```python
from build123d import *

# Parameters (mm, degrees)
F0_R     = 2.5
F1_DEPTH = 5
F2_SIZE  = 4.99999


# Not quite as in the source:
# - a fillet or chamfer is up to 0.001 mm smaller than in the source, because OpenCascade refuses the exact size


with BuildPart() as f1:
    # F0 (on Top) → F1 (new body)
    with BuildSketch(Plane.XY):
        with BuildLine():
            ThreePointArc((100, 15), (97.0710678119, 22.0710678119), (90, 25))
            Line((90, 25), (-90, 25))
            ThreePointArc((-90, 25), (-97.0710678119, 22.0710678119), (-100, 15))
            Line((-100, 15), (-100, -15))
            ThreePointArc((-100, -15), (-97.0710678119, -22.0710678119), (-90, -25))
            Line((-90, -25), (90, -25))
            ThreePointArc((90, -25), (97.0710678119, -22.0710678119), (100, -15))
            Line((100, -15), (100, 15))
        make_face()
        with Locations((-50, 0)):
            Circle(F0_R, mode=Mode.SUBTRACT)
        with Locations((50, 0)):
            Circle(F0_R, mode=Mode.SUBTRACT)
    extrude(amount=F1_DEPTH)

    # F2 (size 5 in the source; OpenCascade refuses exactly that, so slightly less here)
    f2_edges = [f1.edges().sort_by_distance(p)[0] for p in [
        (-52.5, 0, 0),
        (47.5, 0, 0),
    ]]
    chamfer(f2_edges, length=F2_SIZE)


solid = f1.part
```
Source: CAD feature listing. Evaluate the final solid. Frame: model axes, mm. Round coordinates to 2 decimals unless told otherwise and drop trailing zeros. Loops run counter-clockwise (first coordinate to the right, second up) from the corner with the lowest first, then second, coordinate; pieces in that order, holes last. Notation, with made-up numbers: M -36,-11 L 6,-11 A29 cw 6,10 Z; hole C -31.75,-2 d2. An arc over 180 degrees is marked long. Use a Markdown table: item, result. Add a question column.
1. Ray query, line 1 along X through (y, z) = (3, 3.1); line 2 along X through (y, z) = (-4.5, 1.75); line 3 along X through (y, z) = (21.5, 4.8). Return the intervals inside material, ascending. Write a range as [from, to].
2. Cut plane D-D, the plane y = 21. Output: boundary loops of the cut face in (x, z), and give its area (3 significant figures).
3. Pull-direction query (X, two-part tool) for faces 1 (the conical face through (52.68, 0.84, 4.69)), 2 (the flat face through (100, 0, 2)), 3 (the flat face through (-1, 0, 5)); classes: +X half, -X half, draft (parallel to the pull), parting line (faces both ways), or undercut.
4. Cut plane C-C, the plane y = 0. State how many separate pieces and enclosed holes the cut face has, and give its area (3 significant figures).
5. Cut plane B-B, the plane z = 3.45. Output: boundary loops of the cut face in (x, y), and give its area (3 significant figures).
Solution:
| question | item | result |
|---|---|---|
| 1 | line 1 | x = [-100, -53.22], [-46.78, 46.78], [53.22, 100] |
| 1 | line 2 | x = [-100, -53.58], [-46.42, 46.42], [53.58, 100] |
| 1 | line 3 | x = [-97.6, 97.6] |
| 2 | outline | M -98,0 L 98,0 L 98,5 L -98,5 Z |
| 2 | area | 980 mm2 |
| 3 | face 1 | undercut |
| 3 | face 2 | +X half |
| 3 | face 3 | draft |
| 4 | separate pieces | 3 |
| 4 | enclosed holes | 0 |
| 4 | area | 900 mm2 |
| 5 | outline | M -100,-15 A10 ccw -90,-25 L 90,-25 A10 ccw 100,-15 L 100,15 A10 ccw 90,25 L -90,25 A10 ccw -100,15 Z; hole C -50,0 d8.1; hole C 50,0 d8.1 |
| 5 | area | 9,810 mm2 |
